Part model, mm, in its own coordinate system. A direction names the side the tool comes from. Coordinates: 2 decimals unless noted, no trailing zeros. Loops run counter-clockwise (first coordinate to the right, second up) from the corner with the lowest first, then second, coordinate; pieces in that order, holes last. Notation, with made-up numbers: M 8,-4 L 54,-4 A19 cw 54,9 Z; hole C 46.5,68.5 d3. An arc over 180 degrees is marked long. Answer as a JSON object with one key per item and string values. Group by question number.
1. Drill centre lines: L1, parallel to Z at x = 10.5, y = -488.5; L2, parallel to Y at x = 0, z = -632. Where is each one in solid material? Low to high.
2. Saw through at A-A on y = -200. Write the cut outline in (x, z).
3. Mould opens along Y. For faces 1 (the face through (0, 650, -9)), 2 (the face through (0, -9, -650)), 3 (the face through (0, -600, -8)) say: released by +Y, released by -Y, zero draft, split by the parting line, or undercut.
4. 3-axis set-ups, long thin cutter, end or side, ignore diameter. For faces 4 (the face through (0, -650, -9)), 5 (the face through (0, -8, 600)): which of +Z, -Z, +X, -X, +Y, -Y reach the whole face in a straight line?
5. Saw through at C-C on x = -17.5. Write the cut outline in (y, z), then the cut area to 3 significant figures.
from build123d import *

# Parameters (mm, degrees)
SKETCH012_R      = 5
EXTRUDE012_DEPTH = 1500
SKETCH011_W      = 1300
SKETCH011_H      = 1300
SKETCH011_W_2    = 1200
SKETCH011_H_2    = 1200
EXTRUDE011_DEPTH = 25


with BuildPart() as extrude012:
    # Sketch012 (on Face1 of Extrude011) → Extrude012 (new body)
    with BuildSketch(Plane.XY.offset(650)):
        Circle(SKETCH012_R)
    extrude(amount=-EXTRUDE012_DEPTH)


with BuildPart() as cut006:
    # Sketch011 → Extrude011 (new body, symmetric)
    with BuildSketch(Plane.YZ):
        Rectangle(SKETCH011_W, SKETCH011_H)
        Rectangle(SKETCH011_W_2, SKETCH011_H_2, mode=Mode.SUBTRACT)
    extrude(amount=EXTRUDE011_DEPTH, both=True)

    # Cut006: cut Extrude012
    add(extrude012.part, mode=Mode.SUBTRACT)


solid = cut006.part
Outcome:
{
 "1": {"L1": "z = -650 to -600, 600 to 650", "L2": "y = -650 to -5, 5 to 650"},
 "2": {"outline": "M -25,-650 L 25,-650 L 25,-600 L -25,-600 Z; M -25,600 L 25,600 L 25,650 L -25,650 Z"},
 "3": {"face 1": "released by +Y", "face 2": "zero draft", "face 3": "undercut"},
 "4": {"face 4": "+Z, -Z, +X, -X, -Y", "face 5": "+X, -X"},
 "5": {"outline": "M -650,-650 L 650,-650 L 650,650 L -650,650 Z; hole M -600,-600 L 600,-600 L 600,600 L -600,600 Z", "area": "250,000 mm²"}
}
